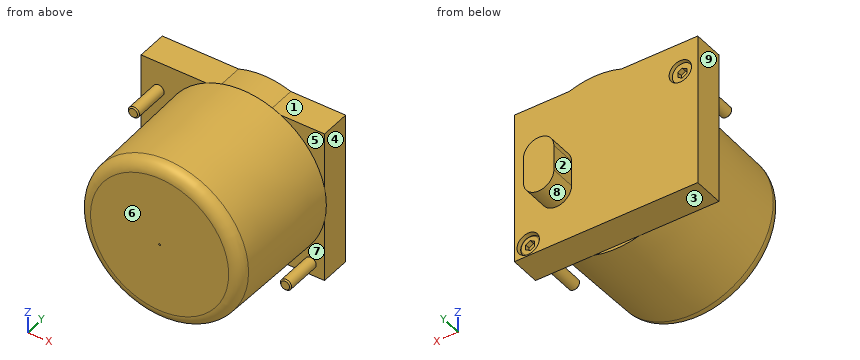
```python
from build123d import *

# Parameters (mm, degrees)
BOSS_EXTRUDE1_DEPTH = 6.8
CUT_EXTRUDE1_DEPTH  = 15
CUT_EXTRUDE2_DEPTH  = 8
BOSS_EXTRUDE2_DEPTH = 5.7
CUT_EXTRUDE3_DEPTH  = 1.1
CUT_EXTRUDE4_DEPTH  = 1.1


with BuildPart() as part:
    # Sketch1 → Revolve1 (revolve)
    with BuildSketch(Plane.XY):
        Polygon((2.4, 0), (19.9, 0), (19.9, -0.858578644), (19.758578644, -1), (18.4, -1), (18.4, -2.5), (19.758578644, -2.5), (19.9, -2.641421356), (19.9, -21), (2.4, -21), align=None)
    revolve(axis=Axis((2.4, -21, 0), (0, 1, 0)))

    # Sketch2 → Boss-Extrude1 (add)
    with BuildSketch(Plane(origin=(0, 0, 0), x_dir=(1, 0, 0), z_dir=(0, 1, 0))):
        with BuildLine():
            Line((-20.5, 17.8), (-20.5, -16.5))
            Line((-20.5, -16.5), (-3.430951895, -16.5))
            ThreePointArc((-3.430951895, -16.5), (2.4, -17.5), (8.230951895, -16.5))
            Line((8.230951895, -16.5), (20.5, -16.5))
            Line((20.5, -16.5), (20.5, 17.8))
            Line((20.5, 17.8), (-20.5, 17.8))
        make_face()
    extrude(amount=BOSS_EXTRUDE1_DEPTH)

    # Sketch3 → Cut-Extrude1 (cut)
    with BuildSketch(Plane(origin=(0, -21, 0), x_dir=(-1, 0, 0), z_dir=(0, -1, 0))):
        with BuildLine():
            Line((0.6, 18.103107468), (0.6, 14.645903864))
            ThreePointArc((0.6, 14.645903864), (-2.4, 14.95), (-5.4, 14.645903864))
            Line((-5.4, 14.645903864), (-5.4, 18.103107468))
            ThreePointArc((-5.4, 18.103107468), (-9.241062733, 17.027106645), (-12.758856756, 15.146504108))
            ThreePointArc((-12.758856756, 15.146504108), (-12.971246379, 10.571246379), (-17.546504108, 10.358856756))
            ThreePointArc((-17.546504108, 10.358856756), (-19.427106645, 6.841062733), (-20.503107468, 3))
            Line((-20.503107468, 3), (-17.045903864, 3))
            ThreePointArc((-17.045903864, 3), (-17.35, 0), (-17.045903864, -3))
            Line((-17.045903864, -3), (-20.503107468, -3))
            ThreePointArc((-20.503107468, -3), (-19.427106645, -6.841062733), (-17.546504108, -10.358856756))
            ThreePointArc((-17.546504108, -10.358856756), (-12.971246379, -10.571246379), (-12.758856756, -15.146504108))
            ThreePointArc((-12.758856756, -15.146504108), (-9.241062733, -17.027106645), (-5.4, -18.103107468))
            Line((-5.4, -18.103107468), (-5.4, -14.645903864))
            ThreePointArc((-5.4, -14.645903864), (-2.4, -14.95), (0.6, -14.645903864))
            Line((0.6, -14.645903864), (0.6, -18.103107468))
            ThreePointArc((0.6, -18.103107468), (4.441062733, -17.027106645), (7.958856756, -15.146504108))
            ThreePointArc((7.958856756, -15.146504108), (8.171246379, -10.571246379), (12.746504108, -10.358856756))
            ThreePointArc((12.746504108, -10.358856756), (14.627106645, -6.841062733), (15.703107468, -3))
            Line((15.703107468, -3), (12.245903864, -3))
            ThreePointArc((12.245903864, -3), (12.55, 0), (12.245903864, 3))
            Line((12.245903864, 3), (15.703107468, 3))
            ThreePointArc((15.703107468, 3), (14.627106645, 6.841062733), (12.746504108, 10.358856756))
            ThreePointArc((12.746504108, 10.358856756), (8.171246379, 10.571246379), (7.958856756, 15.146504108))
            ThreePointArc((7.958856756, 15.146504108), (4.441062733, 17.027106645), (0.6, 18.103107468))
        make_face()
    extrude(amount=-CUT_EXTRUDE1_DEPTH, mode=Mode.SUBTRACT)

    # Sketch4 → Cut-Extrude2 (cut)
    with BuildSketch(Plane(origin=(0, -21, 0), x_dir=(-1, 0, 0), z_dir=(0, -1, 0))):
        Polygon((18.813203436, -14.142135624), (4.671067812, 0), (18.813203436, 14.142135624), (11.742135624, 21.213203436), (-2.4, 7.071067812), (-16.542135624, 21.213203436), (-23.613203436, 14.142135624), (-9.471067812, 0), (-23.613203436, -14.142135624), (-16.542135624, -21.213203436), (-2.4, -7.071067812), (11.742135624, -21.213203436), align=None)
    extrude(amount=-CUT_EXTRUDE2_DEPTH, mode=Mode.SUBTRACT)

    # Sketch5 → Boss-Extrude2 (add)
    with BuildSketch(Plane(origin=(0, 6.8, 0), x_dir=(1, 0, 0), z_dir=(0, 1, 0))):
        with BuildLine():
            Line((14.5, 0.06), (14.5, 5.8))
            ThreePointArc((14.5, 5.8), (11.1, 9.2), (7.7, 5.8))
            Line((7.7, 5.8), (7.7, 0.06))
            ThreePointArc((7.7, 0.06), (11.1, -3.34), (14.5, 0.06))
        make_face()
    extrude(amount=BOSS_EXTRUDE2_DEPTH)

    # Sketch6 → Cut-Revolve1 (revolve, cut)
    with BuildSketch(Plane.XY.offset(-15)):
        Polygon((17.4, 6.8), (19.9, 6.8), (19.9, 3.8), (18.65, 3.8), (18.65, -0.2), (17.4, -0.2), align=None)
    revolve(axis=Axis((17.4, -0.2, -15), (0, 1, 0)), mode=Mode.SUBTRACT)

    # Sketch7 → Revolve2 (revolve)
    with BuildSketch(Plane.XY.offset(-15)):
        with BuildLine():
            Line((17.4, 6.15), (19.4, 6.15))
            ThreePointArc((19.4, 6.15), (19.576776695, 6.076776695), (19.65, 5.9))
            Line((19.65, 5.9), (19.65, 3.8))
            Line((19.65, 3.8), (18.65, 3.8))
            Line((18.65, 3.8), (18.65, -7.924))
            Line((18.65, -7.924), (18.374, -8.2))
            Line((18.374, -8.2), (17.4, -8.2))
            Line((17.4, -8.2), (17.4, 6.15))
        make_face()
    revolve(axis=Axis((17.4, -8.2, -15), (0, 1, 0)))

    # Sketch8 → Cut-Extrude3 (cut)
    with BuildSketch(Plane(origin=(0, 6.15, 0), x_dir=(1, 0, 0), z_dir=(0, 1, 0))):
        Polygon((16.4, 14.422649731), (17.4, 13.845299462), (18.4, 14.422649731), (18.4, 15.577350269), (17.4, 16.154700538), (16.4, 15.577350269), align=None)
    extrude(amount=-CUT_EXTRUDE3_DEPTH, mode=Mode.SUBTRACT)

    # Sketch9 → Cut-Revolve2 (revolve, cut)
    with BuildSketch(Plane.XY.offset(10)):
        Polygon((-16.6, 6.8), (-14.1, 6.8), (-14.1, 3.8), (-15.35, 3.8), (-15.35, -0.2), (-16.6, -0.2), align=None)
    revolve(axis=Axis((-16.6, -0.2, 10), (0, 1, 0)), mode=Mode.SUBTRACT)

    # Sketch10 → Revolve3 (revolve)
    with BuildSketch(Plane.XY.offset(10)):
        Polygon((-16.6, 6.15), (-14.35, 6.15), (-14.35, 3.8), (-15.35, 3.8), (-15.35, -7.924), (-15.626, -8.2), (-16.6, -8.2), align=None)
    revolve(axis=Axis((-16.6, -8.2, 10), (0, 1, 0)))

    # Sketch11 → Cut-Extrude4 (cut)
    with BuildSketch(Plane(origin=(0, 6.15, 0), x_dir=(1, 0, 0), z_dir=(0, 1, 0))):
        Polygon((-17.6, -10.577350269), (-16.6, -11.154700538), (-15.6, -10.577350269), (-15.6, -9.422649731), (-16.6, -8.845299462), (-17.6, -9.422649731), align=None)
    extrude(amount=-CUT_EXTRUDE4_DEPTH, mode=Mode.SUBTRACT)

    # Sketch12 → Revolve4 (revolve)
    with BuildSketch(Plane.XY):
        with BuildLine():
            Line((2.6, -26), (2.6, -27))
            Line((2.6, -27), (17.846723092, -27))
            ThreePointArc((17.846723092, -27), (19.696678603, -26.242917592), (20.485096336, -24.406097884))
            Line((20.485096336, -24.406097884), (20.9, 0))
            Line((20.9, 0), (19.89985551, 0))
            Line((19.89985551, 0), (19.485240806, -24.389100276))
            ThreePointArc((19.485240806, -24.389100276), (18.995607117, -25.529826594), (17.846723028, -26))
            Line((17.846723028, -26), (2.6, -26))
        make_face()
    revolve(axis=Axis((2.4, -27, 0), (0, 1, 0)))


solid = part.part
```
Geometry check sheet. Reference: the model listing, model coordinates, mm. Face numbers are marked on the shaded views. A direction names the side the tool comes from. Give positions to 0.01 mm unless a question says otherwise; leave off trailing zeros. Loops run counter-clockwise (first coordinate to the right, second up) from the corner with the lowest first, then second, coordinate; pieces in that order, holes last. Notation, with made-up numbers: M 33,62.25 L 77,62.25 A18 cw 77,66.25 Z; hole C 3.25,16.5 d1. An arc over 180 degrees is marked long. Write item = value, one per line.
(1) Sectioned sample at B-B, the plane z = -8. State how many separate pieces and enclosed holes the cut face has, plus the area to 3 significant figures.
Answer below:
separate_pieces = 1
enclosed_holes = 3
area = 578 mm2
(2) Release check for a two-part mould opening along X. For the marked faces 6, 7, 8 and 9 record: released by +X, released by -X, zero draft, split by the parting line, or undercut.
Answer below:
face_6 = zero draft
face_7 = undercut
face_8 = split by the parting line
face_9 = released by -X
(3) Sectioned sample at A-A, the plane y = -20. Record the cut outline in (x, z).
Answer below:
outline = C 2.4,0 d36.32; hole M -14.5,-3 A17.16 ccw -0.6,-16.9 L -0.6,-14.65 A14.95 ccw 5.4,-14.65 L 5.4,-16.9 A17.16 ccw 19.3,-3 L 17.05,-3 A14.95 ccw 17.05,3 L 19.3,3 A17.16 ccw 5.4,16.9 L 5.4,14.65 A14.95 ccw -0.6,14.65 L -0.6,16.9 A17.16 ccw -14.5,3 L -12.25,3 A14.95 ccw -12.25,-3 Z
(4) Gauge pin test, flat ends, axial feed: pin 1 Ø10 at (y, z) = (3.5, 7) entering from +X; pin 2 Ø0.7 at (x, y) = (19, -15) entering from +Z; pin 3 Ø0.7 at (y, z) = (-14, 15.5) entering from +X. Record the tip position at first contact, or that the pin passes through.
Answer below:
pin_1 = 20.58
pin_2 = 8.3
pin_3 = 12.6
(5) Material ranges on line 1 (X direction, y = 5, z = -15); line 2 (X direction, y = 5.1, z = -15); line 3 (X direction, y = 4.6, z = 10), recorded low to high. Write a range as [from, to].
Answer below:
line_1 = [-20.5, 14.9], [15.15, 19.65], [19.9, 20.5]
line_2 = [-20.5, 14.9], [15.15, 16.4], [18.4, 19.65], [19.9, 20.5]
line_3 = [-20.5, -19.1], [-18.85, -14.35], [-14.1, 20.5]
(6) Tool access check on the marked faces 1, 2, 3, 4 and 5. Record the directions out of +Z, -Z, +X, -X, +Y, -Y that give a thin tool (end or side, any length) a straight path to the whole face; none if there is none.
Answer below:
face_1 = +Z, +X, +Y
face_2 = +Z, -Z, -X, +Y
face_3 = -Z, +X, -X, +Y
face_4 = +Z, -Z, +X, +Y
face_5 = +Z, +X, -Y
